Design review of the part shown in the three views and the two pictorial views. Dimensions are in mm from the part's minimum x, y and z. A direction names the side the tool comes from. Give positions to 0.01 mm unless a question says otherwise; leave off trailing zeros. Loops run counter-clockwise (first coordinate to the right, second up) from the corner with the lowest first, then second, coordinate; pieces in that order, holes last.
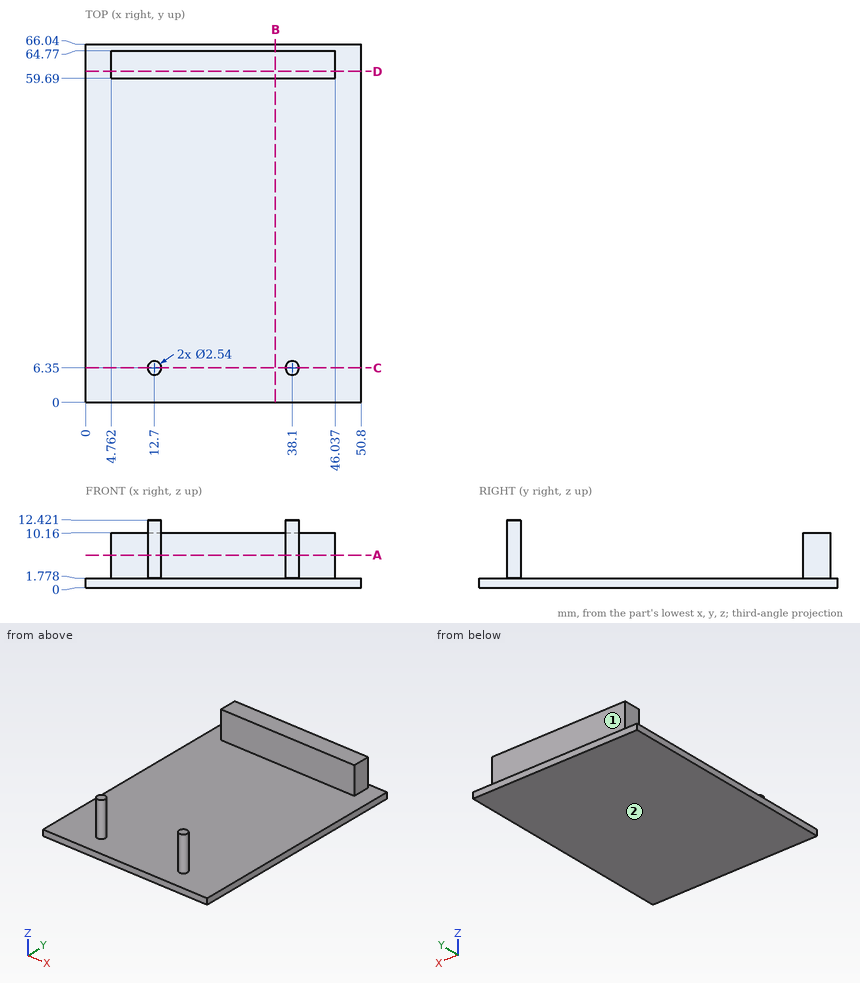
Q1. Take a section at A-A (z = 6). Give the boundary of the cut face in (x, y), plus the area to 3 significant figures.
Results:
outline: (4.76, 59.69) - (46.04, 59.69) - (46.04, 64.77) - (4.76, 64.77) - close; circle Ø2.54 at (12.7, 6.35); circle Ø2.54 at (38.1, 6.35)
area: 220 mm2
Q2. Wall thickness on line 1 (Z direction, x = 23.5, y = 19.5); line 2 (Y direction, x = 44.5, z = 5.25); line 3 (Y direction, x = 12, z = 2.75): over which ranges is each line inside the solid? List them lowest first.
Results:
line 1: z = 0 to 1.78
line 2: y = 59.69 to 64.77
line 3: y = 5.29 to 7.41, 59.69 to 64.77
Q3. Take a section at C-C (y = 6.35). Give the boundary of the cut face in (x, z).
Results:
outline: (0, 0) - (50.8, 0) - (50.8, 1.78) - (39.37, 1.78) - (39.37, 12.42) - (36.83, 12.42) - (36.83, 1.78) - (13.97, 1.78) - (13.97, 12.42) - (11.43, 12.42) - (11.43, 1.78) - (0, 1.78) - close
Q4. Tool access review of the marked faces 1 and 2: name each direction out of +Z, -Z, +X, -X, +Y, -Y from which nothing blocks a thin tool from reaching the whole face with its end or side.
Results:
face 1: +Z, +X, -X, +Y
face 2: -Z, +X, -X, +Y, -Y
Q5. Insertion check: pin 1 (4 mm diameter, centred on x = 17, y = 55, fed in from -Z); pin 2 (2.5 mm diameter, centred on x = 35.5, z = 5.5, fed in from +Y); pin 3 (5.5 mm diameter, centred on y = 63.5, z = 5, fed in from +X); pin 4 (6.5 mm diameter, centred on x = 19.5, z = 7.5, fed in from -Y). Each pin has a flat end and moves straight along its axis. Give the tip position at first contact, or say it passes through.
Results:
pin 1: stops at z = 0
pin 2: stops at y = 64.77
pin 3: stops at x = 46.04
pin 4: stops at y = 59.69
Q6. Take a section at D-D (y = 61). Give the boundary of the cut face in (x, z).
Results:
outline: (0, 0) - (50.8, 0) - (50.8, 1.78) - (46.04, 1.78) - (46.04, 10.16) - (4.76, 10.16) - (4.76, 1.78) - (0, 1.78) - close
Q7. Take a section at B-B (x = 35). Give the boundary of the cut face in (y, z), plus the area to 3 significant figures.
Results:
outline: (0, 0) - (66.04, 0) - (66.04, 1.78) - (64.77, 1.78) - (64.77, 10.16) - (59.69, 10.16) - (59.69, 1.78) - (0, 1.78) - close
area: 160 mm2
